Geometry check sheet. Reference: the model listing, model coordinates, mm. A direction names the side the tool comes from. Give positions to 0.01 mm unless a question says otherwise; leave off trailing zeros. Loops run counter-clockwise (first coordinate to the right, second up) from the corner with the lowest first, then second, coordinate; pieces in that order, holes last.
1. Release check for a two-part mould opening along Y. For faces 1 (the flat face through (0.3, -4.3, -12.739)), 2 (the cylindrical face through (-6, 0, -7)), 3 (the cylindrical face through (-0.651, -7.043, -10.204)), 4 (the flat face through (-1.42, -3.92, -6.739)) record: +Y half, -Y half, draft (parallel to the pull), parting line (faces both ways), or undercut.
2. Cross-section at A-A, the plane z = -10. Record the cut outline in (x, y), plus the area to 3 significant figures.
3. Cross-section at C-C, the plane x = 12. Record the cut outline in (y, z), plus the area to 3 significant figures.
4. Go/stop test with flat-tipped pins: pin 1 Ø3 at (y, z) = (11, -11.5) entering from -X; pin 2 Ø2 at (x, z) = (-11, -11.5) entering from +Y; pin 3 Ø2 at (x, z) = (4.5, -9) entering from -Y. Record where each tip stops, or that it passes through.
5. Material ranges on L1, parallel to X at y = 2, z = -11.75; L2, parallel to Y at x = 3, z = -8.25; L3, parallel to Z at x = -0.5, y = -20.5, recorded low to high.
6. Cross-section at B-B, the plane x = 0. Record the cut outline in (y, z), plus the area to 3 significant figures.
7. Tool access check on faces 5 (the cylindrical face through (17.847, -2.343, -14.711)), 6 (the flat face through (-5, -5, -7.739)), 7 (the cylindrical face through (-0.651, 16.957, -10.204)). Record the directions out of +Z, -Z, +X, -X, +Y, -Y that give a thin tool (end or side, any length) a straight path to the whole face; none if there is none.
from build123d import *

# Parameters (mm, degrees)
SKETCH_2_R          = 5
CUT_EXTRUDE_1_DEPTH = 10
SKETCH_3_R          = 6
SKETCH_3_R_2        = 4
EXTRUDE_1_DEPTH     = 1


with BuildPart() as part:
    # Эскиз1 → Повернуть1 (revolve)
    with BuildSketch(Plane(origin=(0, 0, 0), x_dir=(0, 0, -1), z_dir=(1, 0, 0))):
        Polygon((7.739063178, 4), (7.739063178, 25), (16.739063178, 25), (16.739063178, 18), (12.739063178, 18), (12.739063178, 4), align=None)
    revolve(axis=Axis((0, 0, 0), (0, 0, -1)))

    # Эскиз2 → Вырез-Вытянуть1 (cut, through all)
    with BuildSketch(Plane.XY.offset(-7.739063178)):
        with Locations((0, 12)):
            Circle(SKETCH_2_R)
        with Locations((12, 0)):
            Circle(SKETCH_2_R)
        with Locations((0, -12)):
            Circle(SKETCH_2_R)
        with Locations((-12, 0)):
            Circle(SKETCH_2_R)
    extrude(amount=-CUT_EXTRUDE_1_DEPTH, mode=Mode.SUBTRACT)

    # Эскиз3 → Бобышка-Вытянуть1 (add)
    with BuildSketch(Plane.XY.offset(-7.739063178)):
        Circle(SKETCH_3_R)
        Circle(SKETCH_3_R_2, mode=Mode.SUBTRACT)
    extrude(amount=EXTRUDE_1_DEPTH)


solid = part.part
Result:
1. face 1: undercut
1. face 2: parting line
1. face 3: undercut
1. face 4: draft
2. outline: circle Ø50 at (0, 0); hole circle Ø10 at (-12, 0); hole circle Ø10 at (0, -12); hole circle Ø10 at (0, 12); hole circle Ø8 at (0, 0); hole circle Ø10 at (12, 0)
2. area: 1,600 mm2
3. outline: (-21.93, -16.74) - (-13.42, -16.74) - (-13.42, -12.74) - (-5, -12.74) - (-5, -7.74) - (-21.93, -7.74) - close; (5, -12.74) - (13.42, -12.74) - (13.42, -16.74) - (21.93, -16.74) - (21.93, -7.74) - (5, -7.74) - close
3. area: 237 mm2
4. pin 1: stops at x = -23.12
4. pin 2: stops at y = 22.91
4. pin 3: stops at y = -24.75
5. L1: x = -24.92 to -16.58, -7.42 to -3.46, 3.46 to 7.42, 16.58 to 24.92
5. L2: y = -24.82 to -16, -8 to -2.65, 2.65 to 8, 16 to 24.82
5. L3: z = -16.74 to -7.74
6. outline: (-25, -16.74) - (-18, -16.74) - (-18, -12.74) - (-17, -12.74) - (-17, -7.74) - (-25, -7.74) - close; (-7, -12.74) - (-4, -12.74) - (-4, -6.74) - (-6, -6.74) - (-6, -7.74) - (-7, -7.74) - close; (4, -12.74) - (7, -12.74) - (7, -7.74) - (6, -7.74) - (6, -6.74) - (4, -6.74) - close; (17, -12.74) - (18, -12.74) - (18, -16.74) - (25, -16.74) - (25, -7.74) - (17, -7.74) - close
6. area: 170 mm2
7. face 5: -Z
7. face 6: +Z
7. face 7: +Z, -Z
